The figure shows three views and two pictorial views of one solid part (mm, origin at its lowest corner). Answer the questions. A direction names the side the tool comes from. Round coordinates to 2 decimals unless told otherwise and drop trailing zeros. Write each loop counter-clockwise with the first axis right and the second up, starting at its lowest first coordinate (ties: lowest second). Pieces come first, ordered by that corner, then holes. Notation, with made-up numbers: (55, -34) -> (69, -34) arc R11 cw to (69, -15) -> close; hole circle Ø10 at (79, -11). An arc over 180 degrees is marked (long way). One line per item, written item: value.
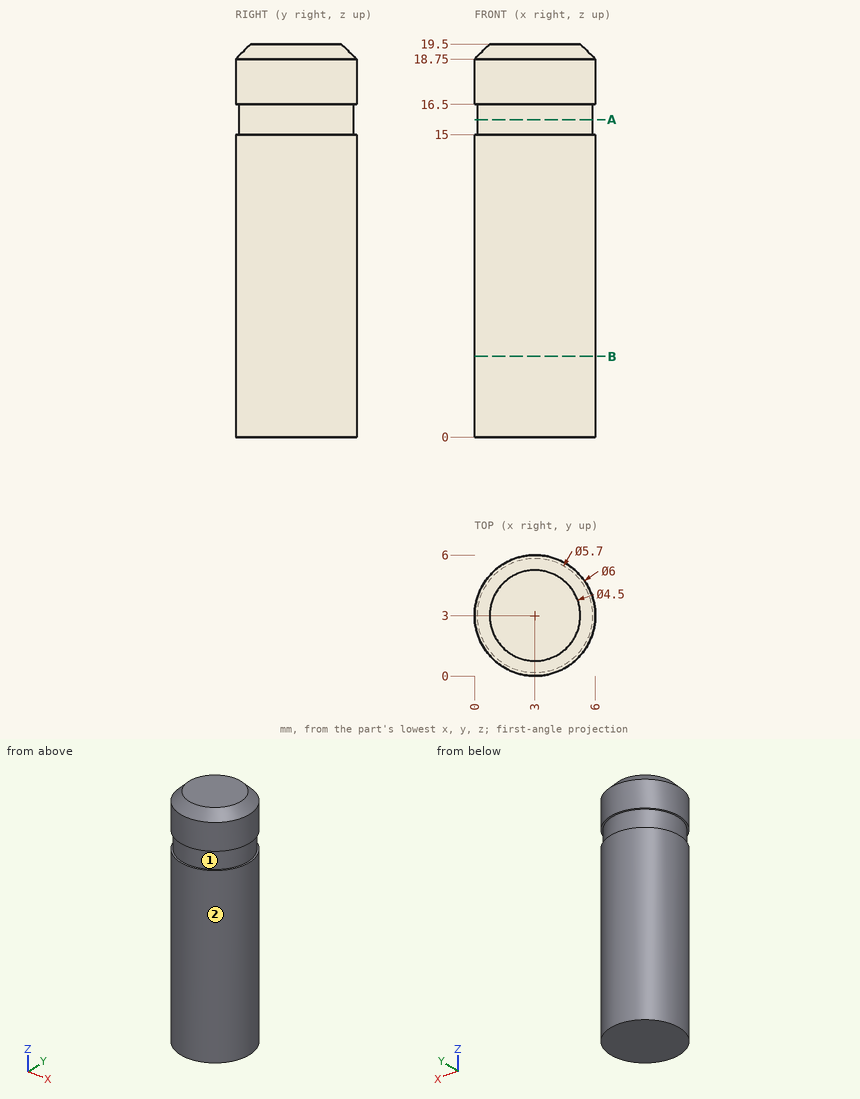
(1) A tool of negligible diameter and unlimited length cuts with its end or side. For the marked faces 1 and 2, from which of +Z, -Z, +X, -X, +Y, -Y can it reach the whole face along a straight path? Write none if from no direction.
Reported:
face 1: none
face 2: +Z, -Z
(2) A flat-ended cylindrical pin translates along its axis: pin 1 Ø1.5 at (y, z) = (1, 2.5) entering from +X. Find the tip coordinate at first contact, or state that the pin passes through.
Reported:
pin 1: stops at x = 5.73
(3) Find section A-A on z = 15.75. Give the vertices of the cut face in (x, y).
Reported:
outline: circle Ø5.7 at (3, 3)
(4) Find section B-B on z = 4. Give the vertices of the cut face in (x, y).
Reported:
outline: circle Ø6 at (3, 3)
(5) Consider probe 1 along X at (y, z) = (2.85, 4.5); probe 2 along X at (y, z) = (3.95, 17.5); probe 3 along Y at (x, z) = (1.15, 18). Determine where each line is inside the solid, lowest interval first.
Reported:
probe 1: x = 0 to 6
probe 2: x = 0.15 to 5.85
probe 3: y = 0.64 to 5.36
